Check sheet for the modelled part. Datum: model origin and axes. Units: mm. Face numbers are marked on the shaded views. Give positions to 0.01 mm unless a question says otherwise; leave off trailing zeros. Order: outer loops, then holes, each group sorted by start corner. A loop starts at its lowest first (then second) coordinate and runs counter-clockwise, first axis right, second up. Notation, with made-up numbers: (60.5, -12.75) -> (110.5, -12.75) arc R30 cw to (110.5, 10.25) -> close; hole circle Ø8 at (-35.5, 63.5). An arc over 180 degrees is marked (long way). Write each question's results on one line, items separated by ' | '.
from build123d import *

# Parameters (mm, degrees)
BOSS_EXTRUDE1_DEPTH = 1.5
BOSS_EXTRUDE4_DEPTH = 8
SKETCH6_W           = 50
SKETCH6_H           = 1
CUT_EXTRUDE1_DEPTH  = 1
SKETCH10_W          = 50
SKETCH10_H          = 1
CUT_EXTRUDE2_DEPTH  = 1
SKETCH11_W          = 50
SKETCH11_H          = 1
CUT_EXTRUDE3_DEPTH  = 1
FILLET1_R           = 1
FILLET2_R           = 0.1


with BuildPart() as part:
    # Sketch2 → Boss-Extrude1 (new body)
    with BuildSketch(Plane(origin=(0, 0, 0), x_dir=(1, 0, 0), z_dir=(0, 1, 0))):
        with BuildLine():
            Line((6, 9.034557534), (6, 0))
            Line((6, 0), (54, 0))
            Line((54, 0), (54, 12.034557534))
            ThreePointArc((54, 12.034557534), (51.454038521, 15), (54, 17.965442466))
            Line((54, 17.965442466), (54, 50))
            Line((54, 50), (6, 50))
            Line((6, 50), (6, 14.965442466))
            ThreePointArc((6, 14.965442466), (7.822155184, 13.954211406), (8.545961479, 12))
            ThreePointArc((8.545961479, 12), (7.822155184, 10.045788594), (6, 9.034557534))
        make_face()
        with BuildLine():
            ThreePointArc((54, 17.965442466), (51.454038521, 15), (54, 12.034557534))
            Line((54, 12.034557534), (54, 13.052219463))
            ThreePointArc((54, 13.052219463), (52.454038521, 15), (54, 16.947780537))
            Line((54, 16.947780537), (54, 17.965442466))
        make_face()
        with BuildLine():
            Line((54, 13.052219463), (54, 12.034557534))
            ThreePointArc((54, 12.034557534), (56.408249927, 12.723806295), (57.454038521, 15))
            ThreePointArc((57.454038521, 15), (56.408249927, 17.276193705), (54, 17.965442466))
            Line((54, 17.965442466), (54, 16.947780537))
            ThreePointArc((54, 16.947780537), (55.697405514, 16.566537111), (56.454038521, 15))
            ThreePointArc((56.454038521, 15), (55.697405514, 13.433462889), (54, 13.052219463))
        make_face()
        with BuildLine():
            ThreePointArc((6, 14.965442466), (2.545961479, 12), (6, 9.034557534))
            Line((6, 9.034557534), (6, 10.052219463))
            ThreePointArc((6, 10.052219463), (3.545961479, 12), (6, 13.947780537))
            Line((6, 13.947780537), (6, 14.965442466))
        make_face()
        with BuildLine():
            Line((6, 10.052219463), (6, 9.034557534))
            ThreePointArc((6, 9.034557534), (7.822155184, 10.045788594), (8.545961479, 12))
            ThreePointArc((8.545961479, 12), (7.822155184, 13.954211406), (6, 14.965442466))
            Line((6, 14.965442466), (6, 13.947780537))
            ThreePointArc((6, 13.947780537), (7.11249859, 13.243366993), (7.545961479, 12))
            ThreePointArc((7.545961479, 12), (7.11249859, 10.756633007), (6, 10.052219463))
        make_face()
    extrude(amount=BOSS_EXTRUDE1_DEPTH)

    # Sketch2<7> → Boss-Extrude4 (add)
    with BuildSketch(Plane(origin=(0, 0, 0), x_dir=(1, 0, 0), z_dir=(0, 1, 0))):
        with BuildLine():
            Line((0, 0), (6, 0))
            Line((6, 0), (6, 9.034557534))
            ThreePointArc((6, 9.034557534), (2.545961479, 12), (6, 14.965442466))
            Line((6, 14.965442466), (6, 50))
            Line((6, 50), (54, 50))
            Line((54, 50), (54, 17.965442466))
            ThreePointArc((54, 17.965442466), (57.454038521, 15), (54, 12.034557534))
            Line((54, 12.034557534), (54, 0))
            Line((54, 0), (60, 0))
            Line((60, 0), (60, 53.896997513))
            Line((60, 53.896997513), (0, 53.896997513))
            Line((0, 53.896997513), (0, 0))
        make_face()
    extrude(amount=BOSS_EXTRUDE4_DEPTH)

    # Sketch6 → Cut-Extrude1 (cut)
    with BuildSketch(Plane(origin=(6, 0, 0), x_dir=(0, 0, -1), z_dir=(1, 0, 0))):
        with Locations((25, 6)):
            Rectangle(SKETCH6_W, SKETCH6_H)
    extrude(amount=-CUT_EXTRUDE1_DEPTH, mode=Mode.SUBTRACT)

    # Sketch10 → Cut-Extrude2 (cut)
    with BuildSketch(Plane.ZY.offset(-54)):
        with Locations((-25, 6)):
            Rectangle(SKETCH10_W, SKETCH10_H)
    extrude(amount=-CUT_EXTRUDE2_DEPTH, mode=Mode.SUBTRACT)

    # Sketch11 → Cut-Extrude3 (cut)
    with BuildSketch(Plane.XY.offset(-50)):
        with Locations((30, 6)):
            Rectangle(SKETCH11_W, SKETCH11_H)
    extrude(amount=-CUT_EXTRUDE3_DEPTH, mode=Mode.SUBTRACT)

    # Fillet1
    fillet1_edges = [part.edges().sort_by_distance(p)[0] for p in [
        (6, 1.5, -4.517278767),
        (6, 1.5, -32.482721233),
        (30, 1.5, -50),
        (54, 1.5, -33.982721233),
        (54, 1.5, -6.017278767),
        (30, 1.5, 0),
        (54, 3.5, 0),
        (6, 3.5, 0),
        (60, 4, -53.896997513),
        (0, 4, -53.896997513),
        (30, 8, -53.896997513),
        (0, 4, 0),
        (60, 4, 0),
        (60, 8, -26.948498756),
        (57, 8, 0),
        (3, 8, 0),
        (0, 8, -26.948498756),
    ]]
    fillet(fillet1_edges, radius=FILLET1_R)

    # Fillet2
    fillet2_edges = [part.edges().sort_by_distance(p)[0] for p in [
        (55, 6.5, -34.474951361),
        (55, 5.5, -6.025048639),
        (55, 6.5, -6.025048639),
        (55, 5.5, -34.474951361),
        (30, 6.5, -51),
        (30, 5.5, -51),
        (5, 6.5, -32.974951361),
        (5, 5.5, -4.525048639),
        (5, 6.5, -4.525048639),
        (5, 5.5, -32.974951361),
    ]]
    fillet(fillet2_edges, radius=FILLET2_R)


solid = part.part
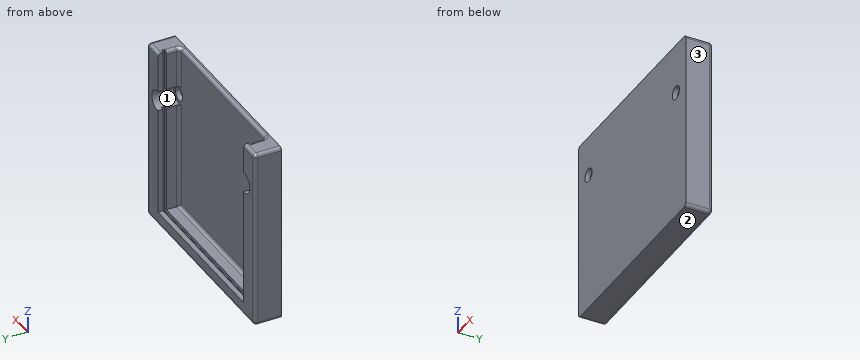
1. Section check B-B on x = 10.5. Record the cut outline in (y, z).
Verdict:
outline: (0, -53.9) -> (7, -53.9) arc R1 ccw to (8, -52.9) -> (8, -50) -> (6.5, -50) -> (6.5, -50.9) arc R0.1 cw to (6.4, -51) -> (5.6, -51) arc R0.1 cw to (5.5, -50.9) -> (5.5, -50) -> (2.5, -50) arc R1 cw to (1.5, -49) -> (1.5, -1) arc R1 ccw to (0.5, 0) -> (0, 0) -> close
2. Material ranges on probe 1 along X at (y, z) = (4.75, -21); probe 2 along X at (y, z) = (6, -27); probe 3 along Y at (x, z) = (5.5, -25.5), recorded low to high. Write a range as from..to.
Verdict:
probe 1: x = 0..6, 54..60 | probe 2: x = 0..5, 55..60 | probe 3: y = 0..5.5, 6.5..8
3. Gauge pin test, flat ends, axial feed: pin 1 Ø5 at (x, z) = (26, -36.5) entering from +Y; pin 2 Ø1 at (x, y) = (27.5, 6.5) entering from +Z. Record the tip position at first contact, or that the pin passes through.
Verdict:
pin 1: stops at y = 1.5 | pin 2: stops at z = -50
4. Section check A-A on z = -32. Record the cut outline in (x, y).
Verdict:
outline: (0, 0) -> (60, 0) -> (60, 7) arc R1 ccw to (59, 8) -> (54, 8) -> (54, 6.5) -> (54.9, 6.5) arc R0.1 cw to (55, 6.4) -> (55, 5.6) arc R0.1 cw to (54.9, 5.5) -> (54, 5.5) -> (54, 2.5) arc R1 cw to (53, 1.5) -> (7, 1.5) arc R1 cw to (6, 2.5) -> (6, 5.5) -> (5.1, 5.5) arc R0.1 cw to (5, 5.6) -> (5, 6.4) arc R0.1 cw to (5.1, 6.5) -> (6, 6.5) -> (6, 8) -> (1, 8) arc R1 ccw to (0, 7) -> close
5. Mould release check, pull along Z, two halves, no side actions. Record for the marked faces 1, 2 and 3: +Z half, -Z half, draft (parallel to the pull), parting line (faces both ways), or undercut.
Verdict:
face 1: undercut | face 2: -Z half | face 3: draft
